```python
from build123d import *

# Parameters (mm, degrees)
SKETCH_R  = 1.7
PAD_DEPTH = 3


with BuildPart() as part:
    # Sketch → Pad (new body)
    with BuildSketch(Plane.XY):
        with BuildLine():
            ThreePointArc((-10.376114, -6.970384), (-10.112712, -7.347316), (-9.835625, -7.714304))
            Line((-9.835625, -7.714304), (-11.441309, -10.027096))
            ThreePointArc((-11.441309, -10.027096), (-11.325129, -11.325129), (-10.027096, -11.441309))
            Line((-10.027096, -11.441309), (-7.714304, -9.835625))
            ThreePointArc((-7.714304, -9.835625), (-7.347316, -10.112712), (-6.970384, -10.376114))
            Line((-6.970384, -10.376114), (-7.782789, -13.071894))
            ThreePointArc((-7.782789, -13.071894), (-7.271181, -14.270495), (-6.000776, -13.979875))
            Line((-6.000776, -13.979875), (-4.297364, -11.738086))
            ThreePointArc((-4.297364, -11.738086), (-3.862712, -11.888206), (-3.422833, -12.022238))
            Line((-3.422833, -12.022238), (-3.362435, -14.837123))
            ThreePointArc((-3.362435, -14.837123), (-2.505478, -15.818966), (-1.387058, -15.149992))
            Line((-1.387058, -15.149992), (-0.459768, -12.491542))
            ThreePointArc((-0.459768, -12.491542), (0, -12.5), (0.459768, -12.491542))
            Line((0.459768, -12.491542), (1.387058, -15.149992))
            ThreePointArc((1.387058, -15.149992), (2.505478, -15.818966), (3.362435, -14.837123))
            Line((3.362435, -14.837123), (3.422833, -12.022238))
            ThreePointArc((3.422833, -12.022238), (7.799066, -9.76855), (10.965856, -6))
            Line((30.259157, -5), (10.965856, -6))
            ThreePointArc((30.259157, -5), (35.006712, 0), (30.259157, 5))
            Line((10.965856, 6), (30.259157, 5))
            ThreePointArc((10.965856, 6), (-1.392635, 12.42218), (-12.022238, 3.422833))
            Line((-12.022238, 3.422833), (-14.837123, 3.362435))
            ThreePointArc((-14.837123, 3.362435), (-15.818966, 2.505478), (-15.149992, 1.387058))
            Line((-15.149992, 1.387058), (-12.491542, 0.459768))
            ThreePointArc((-12.491542, 0.459768), (-12.5, 0), (-12.491542, -0.459768))
            Line((-12.491542, -0.459768), (-15.149992, -1.387058))
            ThreePointArc((-15.149992, -1.387058), (-15.818966, -2.505478), (-14.837123, -3.362435))
            Line((-14.837123, -3.362435), (-12.022238, -3.422833))
            ThreePointArc((-12.022238, -3.422833), (-11.888206, -3.862712), (-11.738086, -4.297364))
            Line((-11.738086, -4.297364), (-13.979875, -6.000776))
            ThreePointArc((-13.979875, -6.000776), (-14.270495, -7.271181), (-13.071894, -7.782789))
            Line((-13.071894, -7.782789), (-10.376114, -6.970384))
        make_face()
        Circle(SKETCH_R, mode=Mode.SUBTRACT)
        with Locations((7, 0)):
            Circle(SKETCH_R, mode=Mode.SUBTRACT)
        with Locations((-7, 0)):
            Circle(SKETCH_R, mode=Mode.SUBTRACT)
        with Locations((30, 0)):
            Circle(SKETCH_R, mode=Mode.SUBTRACT)
    extrude(amount=PAD_DEPTH)


solid = part.part
```
The listing builds one solid part. Answer for the finished solid, in the listing's coordinates (mm). A direction names the side the tool comes from. Give positions to 0.01 mm unless a question says otherwise; leave off trailing zeros. Order: outer loops, then holes, each group sorted by start corner. A loop starts at its lowest first (then second) coordinate and runs counter-clockwise, first axis right, second up.
1) Consider line 1 along Y through (x, z) = (0, 0.65); line 2 along Y through (x, z) = (7, 2.1); line 3 along X through (y, z) = (2, 2.85). Determine where each line is inside the solid, lowest interval first.
Reported:
line 1: y = -12.5 to -1.7, 1.7 to 12.5
line 2: y = -10.36 to -1.7, 1.7 to 10.36
line 3: x = -15.77 to 34.59
2) Find section C-C on y = 7.5. Write down the section's boundary in (x, z), then the cut area to 3 significant figures.
Reported:
outline: (-10, 0) - (10, 0) - (10, 3) - (-10, 3) - close
area: 60.0 mm2
3) Find section A-A on x = 7. Write down the section's boundary in (y, z).
Reported:
outline: (-10.36, 0) - (-1.7, 0) - (-1.7, 3) - (-10.36, 3) - close; (1.7, 0) - (10.36, 0) - (10.36, 3) - (1.7, 3) - close
4) Given P1, Ø1.5, axis at x = 5, z = 2.5, coming from the -Y side; P2, Ø1, axis at y = -10, z = 1, coming from the -X side; P3, Ø1.5, axis at x = 28.5, z = 2, coming from the +Y side, each flat-ended and moving along its own axis, determine where each tip first touches the part or whether it passes through.
Reported:
P1: stops at y = -11.76
P2: stops at x = -11.62
P3: stops at y = 5.13
5) Find section B-B on z = 0.6. Give the number of separate pieces and of enclosed holes in the cut face, then the cut area to 3 significant figures.
Reported:
separate pieces: 1
enclosed holes: 4
area: 747 mm2
6) For faces 5 (the face through (-13.84, 0.93, 1.48)), 6 (the face through (-3.869, -11.886, 1.479)), 7 (the face through (-11.74, -7.38, 1.48)), determine the directions among +Z, -Z, +X, -X, +Y, -Y from which every point of the face is accessible in a straight line to the end or side of a thin tool.
Reported:
face 5: +Z, -Z, -X
face 6: +Z, -Z, -Y
face 7: +Z, -Z
7) Determine the mould class of faces 1 (the face through (-12.843, -5.137, 1.479)), 2 (the face through (7.745, -9.812, 1.479)), 3 (the face through (9, -1, 3)), 4 (the face through (-10.627, -8.855, 1.479)) for opening direction Y: pulls with the +Y half, pulls with the -Y half, needs draft (parallel to the pull), parting line crosses it, or undercut.
Reported:
face 1: undercut
face 2: pulls with the -Y half
face 3: needs draft
face 4: undercut
8) Find section D-D on x = 31. Write down the section's boundary in (y, z), then the cut area to 3 significant figures.
Reported:
outline: (-4.91, 0) - (-1.37, 0) - (-1.37, 3) - (-4.91, 3) - close; (1.37, 0) - (4.91, 0) - (4.91, 3) - (1.37, 3) - close
area: 21.2 mm2
